```python
from build123d import *

# Parameters (mm, degrees)
SKETCH_2_R          = 8
EXTRUDE_1_DEPTH     = 22.9
SKETCH_4_R          = 10.68097998
EXTRUDE_3_DEPTH     = 2
CHAMFER_1_SIZE      = 0.5
CHAMFER_1_SIZE2     = 1.37373871
CHAMFER_2_SIZE      = 0.5
CHAMFER_2_SIZE2     = 1.37373871
CUT_EXTRUDE_1_DEPTH = 2
CUT_EXTRUDE_2_DEPTH = 0.1
SKETCH_9_W          = 0.6
SKETCH_9_H          = 8


with BuildPart() as part:
    # 草图2 → 凸台-拉伸1 (new body)
    with BuildSketch(Plane(origin=(0, 0, 0), x_dir=(1, 0, 0), z_dir=(0, 1, 0))):
        with Locations(Location((0, 0, 0), (0, 0, 270))):
            Circle(SKETCH_2_R)
    extrude(amount=EXTRUDE_1_DEPTH)

    # 草图4 → 凸台-拉伸3 (add)
    with BuildSketch(Plane.XZ):
        with Locations(Location((0, 0, 0), (0, 0, 270))):
            Circle(SKETCH_4_R)
    extrude(amount=-EXTRUDE_3_DEPTH)

    # 倒角1
    chamfer_1_edges = [part.edges().sort_by_distance(p)[0] for p in [
        (0, 0, 10.68097998),
    ]]
    chamfer_1_side = [part.faces().sort_by_distance(p)[0] for p in [
        (0, 1, 10.68097998),
    ]]
    chamfer(chamfer_1_edges, length=CHAMFER_1_SIZE, length2=CHAMFER_1_SIZE2, reference=chamfer_1_side[0])

    # 倒角2
    chamfer_2_edges = [part.edges().sort_by_distance(p)[0] for p in [
        (0, 2, 10.68097998),
    ]]
    chamfer_2_side = [part.faces().sort_by_distance(p)[0] for p in [
        (0, 1.25, 10.68097998),
    ]]
    chamfer(chamfer_2_edges, length=CHAMFER_2_SIZE, length2=CHAMFER_2_SIZE2, reference=chamfer_2_side[0])

    # 草图1 → 切除-拉伸1 (cut)
    with BuildSketch(Plane(origin=(0, 0, 0), x_dir=(1, 0, 0), z_dir=(0, 1, 0))):
        with BuildLine():
            Line((5.34048999, 9.25), (10.68097998, 0))
            ThreePointArc((10.68097998, 0), (9.25, 5.34048999), (5.34048999, 9.25))
        make_face()
        with BuildLine():
            Line((-5.34048999, 9.25), (5.34048999, 9.25))
            ThreePointArc((5.34048999, 9.25), (0, 10.68097998), (-5.34048999, 9.25))
        make_face()
        with BuildLine():
            ThreePointArc((5.34048999, -9.25), (9.25, -5.34048999), (10.68097998, 0))
            Line((10.68097998, 0), (5.34048999, -9.25))
        make_face()
        with BuildLine():
            ThreePointArc((-5.34048999, -9.25), (0, -10.68097998), (5.34048999, -9.25))
            Line((5.34048999, -9.25), (-5.34048999, -9.25))
        make_face()
        with BuildLine():
            ThreePointArc((-10.68097998, 0), (-9.25, -5.34048999), (-5.34048999, -9.25))
            Line((-5.34048999, -9.25), (-10.68097998, 0))
        make_face()
        with BuildLine():
            Line((-10.68097998, 0), (-5.34048999, 9.25))
            ThreePointArc((-5.34048999, 9.25), (-9.25, 5.34048999), (-10.68097998, 0))
        make_face()
    extrude(amount=CUT_EXTRUDE_1_DEPTH, mode=Mode.SUBTRACT)

    # 草图6 → 旋转1 (revolve)
    with BuildSketch(Plane.XY, mode=Mode.PRIVATE) as revolve_1_sk:
        with BuildLine():
            Line((0, 0), (9, 0))
            ThreePointArc((9, 0), (9.4, -0.4), (9, -0.8))
            Line((9, -0.8), (0, -0.8))
            Line((0, -0.8), (0, 0))
        make_face()
    revolve(revolve_1_sk.sketch.rotate(Axis((0, 0, 0), (0, -1, 0)), 270), axis=Axis((0, 0, 0), (0, -1, 0)))

    # 草图7 → 旋转2 (revolve)
    with BuildSketch(Plane.XY, mode=Mode.PRIVATE) as revolve_2_sk:
        with BuildLine():
            Line((0, -0.8), (10.6, -0.8))
            ThreePointArc((10.6, -0.8), (10.69701425, -0.875746437), (10.647058824, -0.988235294))
            Line((10.647058824, -0.988235294), (8.441176471, -2.164705882))
            ThreePointArc((8.441176471, -2.164705882), (7.98507125, -2.340285), (7.5, -2.4))
            Line((7.5, -2.4), (0, -2.4))
            Line((0, -2.4), (0, -0.8))
        make_face()
    revolve(revolve_2_sk.sketch.rotate(Axis((0, -2.4, 0), (0, 1, 0)), 90), axis=Axis((0, -2.4, 0), (0, 1, 0)))

    # 草图8 → 切除-拉伸2 (cut)
    with BuildSketch(Plane.XZ.offset(2.4)):
        with BuildLine():
            Line((-0.5, 2.169099871), (-0.5, 5.169099871))
            ThreePointArc((-0.5, 5.169099871), (0, 5.669099871), (0.5, 5.169099871))
            Line((0.5, 5.169099871), (0.5, 2.169099871))
            ThreePointArc((0.5, 2.169099871), (0, 1.669099871), (-0.5, 2.169099871))
        make_face()
        with BuildLine():
            ThreePointArc((-4.363636364, 4.11809151), (0, -6), (4.363636364, 4.11809151))
            ThreePointArc((4.363636364, 4.11809151), (3.656825707, 4.138553581), (3.636363636, 3.431742925))
            ThreePointArc((3.636363636, 3.431742925), (0, -5), (-3.636363636, 3.431742925))
            ThreePointArc((-3.636363636, 3.431742925), (-3.656825707, 4.138553581), (-4.363636364, 4.11809151))
        make_face()
    extrude(amount=-CUT_EXTRUDE_2_DEPTH, mode=Mode.SUBTRACT)

    # 草图9 → 切除-旋转1 (revolve, cut)
    with BuildSketch(Plane.XY, mode=Mode.PRIVATE) as cut_revolve_1_sk:
        with Locations((7.7, 18.9)):
            Rectangle(SKETCH_9_W, SKETCH_9_H)
    revolve(cut_revolve_1_sk.sketch.rotate(Axis((0, 0, 0), (0, 1, 0)), 90), axis=Axis((0, 0, 0), (0, 1, 0)), mode=Mode.SUBTRACT)

    # 草图10 → 旋转4 (revolve)
    with BuildSketch(Plane.XY, mode=Mode.PRIVATE) as revolve_4_sk:
        Polygon((4.153927956, 22.9), (4.653927956, 22.9), (4.653927956, 24.9), (5.353927956, 24.9), (5.353927956, 25.9), (4.153927956, 25.9), align=None)
    revolve_4 = revolve(revolve_4_sk.sketch.rotate(Axis((4.153927956, 22.9, 0), (0, 1, 0)), 90), axis=Axis((4.153927956, 22.9, 0), (0, 1, 0)))

    # 镜向1: 旋转4 across plane
    add(revolve_4.mirror(Plane(origin=(0, 0, 0), x_dir=(0, 0, 1), z_dir=(1, 0, 0))))


solid = part.part
```
Part model, mm, in its own coordinate system. A direction names the side the tool comes from. Round coordinates to 2 decimals unless told otherwise and drop trailing zeros. Loops run counter-clockwise (first coordinate to the right, second up) from the corner with the lowest first, then second, coordinate; pieces in that order, holes last. Notation, with made-up numbers: (-25, 75.5) -> (28, 75.5) arc R26 cw to (28, 106.5) -> close; hole circle Ø7 at (45, -11.75). An arc over 180 degrees is marked (long way). Use a Markdown table: item, result.
1) Drop flat-ended pins along their axis: pin 1 Ø1.6 at (x, y) = (1, 1) entering from +Z; pin 2 Ø4 at (y, z) = (9.5, 8.5) entering from +X; pin 3 Ø1.5 at (x, y) = (-1, 9) entering from -Z. Give the stop position or say it passes through.
The answers:
| item | result |
|---|---|
| pin 1 | stops at z = 9.25 |
| pin 2 | stops at x = 4.66 |
| pin 3 | stops at z = -8 |
2) Pull direction X, two halves, no side cores. Call faces 5 (the flat face through (-4, 25.9, 0)), 6 (the conical face through (4.888, 1.865, 8.354)), 7 (the cylindrical face through (-4.64, 23.91, 0.11)): pulls with the +X half, pulls with the -X half, needs draft (parallel to the pull), parting line crosses it, or undercut.
The answers:
| item | result |
|---|---|
| face 5 | needs draft |
| face 6 | pulls with the +X half |
| face 7 | undercut |
3) Probe line 1 (Z direction, x = -5.75, y = 15.75); line 2 (Y direction, x = 5.75, z = 0.25); line 3 (Y direction, x = 2.75, z = 6). List the from-to ranges inside material, lowest first. Write a range as [from, to].
The answers:
| item | result |
|---|---|
| line 1 | z = [-4.66, 4.66] |
| line 2 | y = [-2.3, 22.9] |
| line 3 | y = [-2.4, 22.9] |
4) Cut at C-C, the plane y = 12. List the corners of the cut face in (x, z), and give its area (3 significant figures).
The answers:
| item | result |
|---|---|
| outline | circle Ø16 at (0, 0) |
| area | 201 mm2 |
5) Tool access for faces 1 (the flat face through (0, 1, 9.25)), 2 (the flat face through (8, -0.8, -5)), 3 (the flat face through (-8.05, 0.99, -4.56)), 4 (the cylindrical face through (-7.81, 8.36, -1.73)): list every direction of +Z, -Z, +X, -X, +Y, -Y with a clear straight run to the whole face (end or side of a thin tool).
The answers:
| item | result |
|---|---|
| face 1 | +Z, +X, -X, +Y |
| face 2 | none |
| face 3 | -Z, -X, +Y |
| face 4 | +Y |
6) Cut at B-B, the plane y = 15.25. List the corners of the cut face in (x, z).
The answers:
| item | result |
|---|---|
| outline | circle Ø14.8 at (0, 0) |
